from build123d import *

# Parameters (mm, degrees)
F0_W     = 44.90128
F0_H     = 44.90128
F0_R     = 1.6383
F0_R_2   = 3.175
F1_DEPTH = 12.7


with BuildPart() as f1:
    # F0 (on Right) → F1 (new body, symmetric)
    with BuildSketch(Plane.YZ):
        Rectangle(F0_W, F0_H)
        with Locations((-12.714292, -7.3406)):
            Circle(F0_R, mode=Mode.SUBTRACT)
        with Locations((0, -14.6812)):
            Circle(F0_R, mode=Mode.SUBTRACT)
        with Locations((12.714292, -7.3406)):
            Circle(F0_R, mode=Mode.SUBTRACT)
        with Locations((-12.714292, 7.3406)):
            Circle(F0_R, mode=Mode.SUBTRACT)
        Circle(F0_R_2, mode=Mode.SUBTRACT)
        with Locations((12.714292, 7.3406)):
            Circle(F0_R, mode=Mode.SUBTRACT)
        with Locations((0, 14.6812)):
            Circle(F0_R, mode=Mode.SUBTRACT)
    extrude(amount=F1_DEPTH, both=True)


solid = f1.part
For this review, take the finished solid that the model builds, in its own axes (mm). Give positions to 0.01 mm unless a question says otherwise; leave off trailing zeros. Loops run counter-clockwise (first coordinate to the right, second up) from the corner with the lowest first, then second, coordinate; pieces in that order, holes last. Notation, with made-up numbers: (83, 47.25) -> (97, 47.25) arc R25 cw to (97, 73.25) -> close; hole circle Ø10 at (76.25, -3). An arc over 180 degrees is marked (long way). One line per question, with ' | ' between items.
1) To check wall thickness, follow probe 1 along Z at (x, y) = (6.5, 0) (1 decimal); probe 2 along Y at (x, z) = (4.5, 7.5); probe 3 along Z at (x, y) = (-7.25, 12.5). State the ranges of each line that lie inside material, in increasing order.
Resolved:
probe 1: z = -22.5 to -16.3, -13 to -3.2, 3.2 to 13, 16.3 to 22.5 | probe 2: y = -22.45 to -14.34, -11.08 to 11.08, 14.34 to 22.45 | probe 3: z = -22.45 to -8.96, -5.72 to 5.72, 8.96 to 22.45
2) The part is to be moulded in two halves that separate along Y. For faces 1 (the cylindrical face through (-0.18, -13.07, 5.74)), 2 (the flat face through (-12.7, 0, 5)), 3 (the flat face through (0, -22.451, 0)), say which applies: +Y half, -Y half, draft (parallel to the pull), parting line (faces both ways), or undercut.
Resolved:
face 1: undercut | face 2: draft | face 3: -Y half
3) We need section A-A (y = 0). Write out the cut boundary in (x, z) (1 decimal), plus the area to 3 significant figures.
Resolved:
outline: (-12.7, -22.5) -> (12.7, -22.5) -> (12.7, -16.3) -> (-12.7, -16.3) -> close; (-12.7, -13) -> (12.7, -13) -> (12.7, -3.2) -> (-12.7, -3.2) -> close; (-12.7, 3.2) -> (12.7, 3.2) -> (12.7, 13) -> (-12.7, 13) -> close; (-12.7, 16.3) -> (12.7, 16.3) -> (12.7, 22.5) -> (-12.7, 22.5) -> close | area: 813 mm2
4) Insertion check: pin 1 Ø5.5 at (y, z) = (0, 0) entering from -X. The pin has a flat end and moves straight along its axis. Give the tip position at first contact, or say it passes through.
Resolved:
pin 1: passes through
5) We need section C-C (x = -9.5). Write out the cut boundary in (y, z) (3 decimals).
Resolved:
outline: (-22.451, -22.451) -> (22.451, -22.451) -> (22.451, 22.451) -> (-22.451, 22.451) -> close; hole circle Ø3.277 at (-12.714, -7.341); hole circle Ø3.277 at (-12.714, 7.341); hole circle Ø6.35 at (0, 0); hole circle Ø3.277 at (0, -14.681); hole circle Ø3.277 at (0, 14.681); hole circle Ø3.277 at (12.714, -7.341); hole circle Ø3.277 at (12.714, 7.341)
6) We need section B-B (z = 0). Write out the cut boundary in (x, y) (3 decimals), plus the area to 3 significant figures.
Resolved:
outline: (-12.7, -22.451) -> (12.7, -22.451) -> (12.7, -3.175) -> (-12.7, -3.175) -> close; (-12.7, 3.175) -> (12.7, 3.175) -> (12.7, 22.451) -> (-12.7, 22.451) -> close | area: 979 mm2
7) We need section D-D (z = 6.5). Write out the cut boundary in (x, y).
Resolved:
outline: (-12.7, -22.45) -> (12.7, -22.45) -> (12.7, -14.12) -> (-12.7, -14.12) -> close; (-12.7, -11.31) -> (12.7, -11.31) -> (12.7, 11.31) -> (-12.7, 11.31) -> close; (-12.7, 14.12) -> (12.7, 14.12) -> (12.7, 22.45) -> (-12.7, 22.45) -> close
